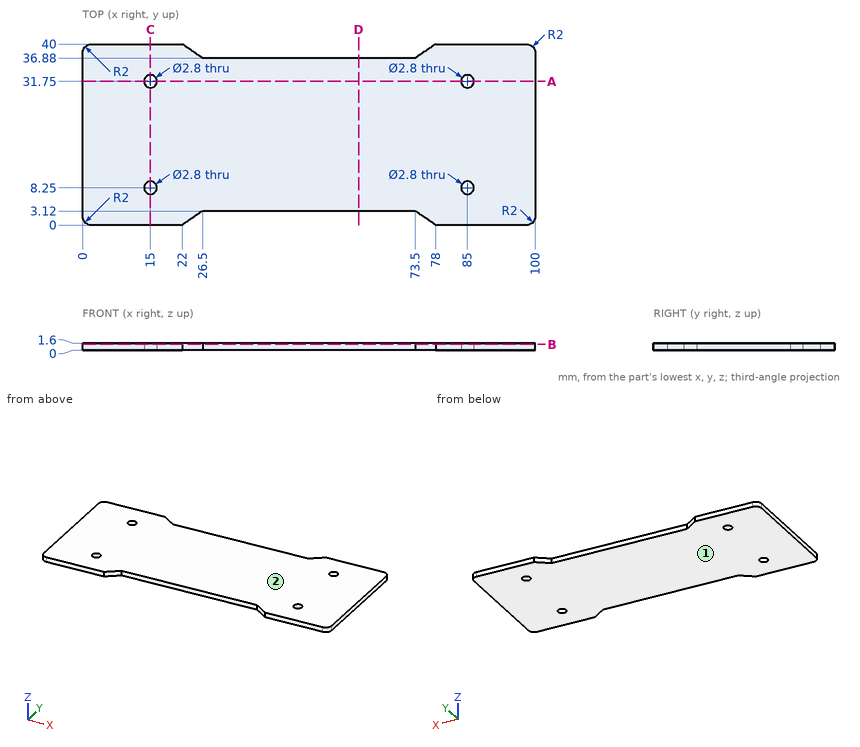
Can you work these out from the drawing? Everything is in mm from the part's minimum corner. Coordinates: 2 decimals unless noted, no trailing zeros. Write each loop counter-clockwise with the first axis right and the second up, starting at its lowest first coordinate (ties: lowest second). Pieces come first, ordered by that corner, then holes. Notation, with made-up numbers: (25, -20) - (81, -20) arc R21 cw to (81, 3) - close; hole circle Ø5 at (86, 0). An arc over 180 degrees is marked (long way). One line per item, written item: value.
1) Suppose I cut it at D-D on x = 61. Write out the boundary of the cut face in (y, z), and give its area (3 significant figures).
Model answer:
outline: (3.12, 0) - (36.88, 0) - (36.88, 1.6) - (3.12, 1.6) - close
area: 54.0 mm²
2) We'd pull the mould along Z, two halves only. Please class the marked faces 1 and 2: pulls with the +Z half, pulls with the -Z half, needs draft (parallel to the pull), parting line crosses it, or undercut.
Model answer:
face 1: pulls with the -Z half
face 2: pulls with the +Z half
3) Suppose I cut it at A-A on y = 31.75. Write out the boundary of the cut face in (x, z), and give its area (3 significant figures).
Model answer:
outline: (0, 0) - (13.6, 0) - (13.6, 1.6) - (0, 1.6) - close; (16.4, 0) - (83.6, 0) - (83.6, 1.6) - (16.4, 1.6) - close; (86.4, 0) - (100, 0) - (100, 1.6) - (86.4, 1.6) - close
area: 151 mm²
4) I need wall thicknesses on line 1 along Y through (x, z) = (85, 0.4); line 2 along X through (y, z) = (32, 0.95); line 3 along X through (y, z) = (7.5, 0.3). Which ranges of each line are inside material? Lowest first, please.
Model answer:
line 1: y = 0 to 6.85, 9.65 to 30.35, 33.15 to 40
line 2: x = 0 to 13.62, 16.38 to 83.62, 86.38 to 100
line 3: x = 0 to 13.82, 16.18 to 83.82, 86.18 to 100
5) Suppose I cut it at B-B on z = 1.35. Write out the boundary of the cut face in (x, y), and give its area (3 significant figures).
Model answer:
outline: (0, 2) arc R2 ccw to (2, 0) - (22, 0) - (26.5, 3.12) - (73.5, 3.12) - (78, 0) - (98, 0) arc R2 ccw to (100, 2) - (100, 38) arc R2 ccw to (98, 40) - (78, 40) - (73.5, 36.88) - (26.5, 36.88) - (22, 40) - (2, 40) arc R2 ccw to (0, 38) - close; hole circle Ø2.8 at (15, 8.25); hole circle Ø2.8 at (15, 31.75); hole circle Ø2.8 at (85, 8.25); hole circle Ø2.8 at (85, 31.75)
area: 3,650 mm²
6) Suppose I cut it at C-C on x = 15. Write out the boundary of the cut face in (y, z).
Model answer:
outline: (0, 0) - (6.85, 0) - (6.85, 1.6) - (0, 1.6) - close; (9.65, 0) - (30.35, 0) - (30.35, 1.6) - (9.65, 1.6) - close; (33.15, 0) - (40, 0) - (40, 1.6) - (33.15, 1.6) - close
7) I'm going to push flat-ended pins straight in: P1, Ø4.5, axis at x = 15, y = 8.25, coming from the +Z side; P2, Ø0.5, axis at x = 47.5, z = 1, coming from the -Y side; P3, Ø0.5, axis at x = 40.5, z = 1, coming from the +Y side. Where does each tip first touch, or does it pass through?
Model answer:
P1: stops at z = 1.6
P2: stops at y = 3.12
P3: stops at y = 36.88
